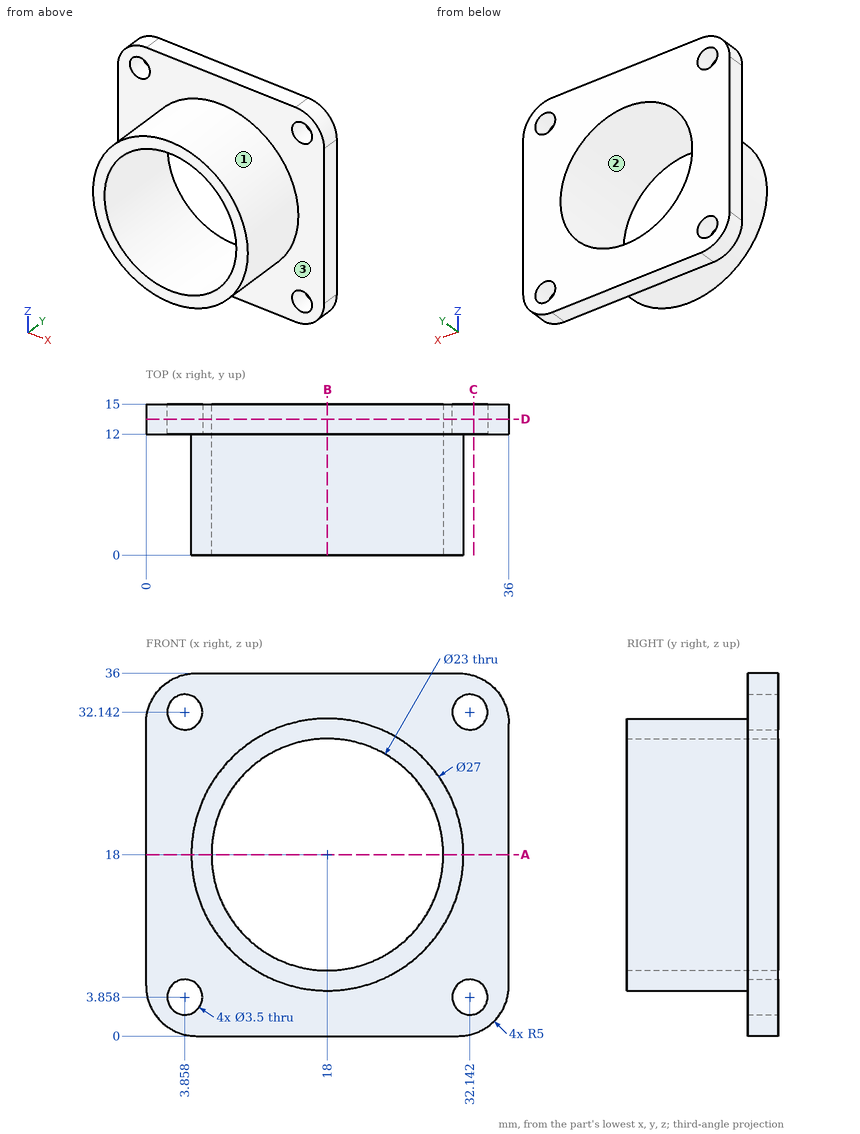
Here's the drawing with two shaded views (mm, measured from the low corner). I have some questions. Round coordinates to 2 decimals unless told otherwise and drop trailing zeros. Order: outer loops, then holes, each group sorted by start corner. A loop starts at its lowest first (then second) coordinate and runs counter-clockwise, first axis right, second up. Notation, with made-up numbers: M 39,9.5 L 72,9.5 A30 ccw 72,37.5 Z; hole C 69,6 d7. An arc over 180 degrees is marked long. Use CSV: the item, a comma, the result in double quotes.
1) I'm going to push flat-ended pins straight in: P1, Ø3, axis at x = 17, y = 8.5, coming from the -Z side; P2, Ø20.5, axis at x = 18, z = 18, coming from the -Y side; P3, Ø6, axis at x = 30, y = 2, coming from the +Z side. Where does each tip first touch, or does it pass through?
Taken from the geometry:
P1,"z = 4.5"
P2,"through"
P3,"z = 28.06"
2) I want a section at B-B (x = 18). List the corners of the cut face in (y, z) for me, then the cut area to 3 significant figures.
Taken from the geometry:
outline,"M 0,4.5 L 12,4.5 L 12,0 L 15,0 L 15,6.5 L 0,6.5 Z; M 0,29.5 L 15,29.5 L 15,36 L 12,36 L 12,31.5 L 0,31.5 Z"
area,"87.0 mm^2"
3) I need wall thicknesses on line 1 along Y through (x, z) = (3.5, 7); line 2 along Z through (x, y) = (3, 13); line 3 along X through (y, z) = (13.25, 10). Which ranges of each line are inside material? Lowest first, please. Write a range as [from, to].
Taken from the geometry:
line 1,"[12, 15]"
line 2,"[0.42, 2.33], [5.38, 30.62], [33.67, 35.58]"
line 3,"[0, 9.74], [26.26, 36]"
4) If we mould it in two halves opening along X, with no side actions, what happens to the marked faces 1, 2 and 3? For each: pulls with the +X half, pulls with the -X half, needs draft (parallel to the pull), parting line crosses it, or undercut.
Taken from the geometry:
face 1,"parting line crosses it"
face 2,"undercut"
face 3,"needs draft"
5) I want a section at A-A (z = 18). List the corners of the cut face in (x, y) for me, then the cut area to 3 significant figures.
Taken from the geometry:
outline,"M 0,12 L 4.5,12 L 4.5,0 L 6.5,0 L 6.5,15 L 0,15 Z; M 29.5,0 L 31.5,0 L 31.5,12 L 36,12 L 36,15 L 29.5,15 Z"
area,"87.0 mm^2"
6) I want a section at C-C (x = 32.5). List the corners of the cut face in (y, z) for me (1 decimal).
Taken from the geometry:
outline,"M 12,0.2 L 15,0.2 L 15,2.1 L 12,2.1 Z; M 12,5.6 L 15,5.6 L 15,30.4 L 12,30.4 Z; M 12,33.9 L 15,33.9 L 15,35.8 L 12,35.8 Z"
7) I want a section at D-D (y = 13.5). List the corners of the cut face in (x, z) for me, then the cut area to 3 significant figures.
Taken from the geometry:
outline,"M 0,5 A5 ccw 5,0 L 31,0 A5 ccw 36,5 L 36,31 A5 ccw 31,36 L 5,36 A5 ccw 0,31 Z; hole C 3.86,3.86 d3.5; hole C 3.86,32.14 d3.5; hole C 18,18 d23; hole C 32.14,3.86 d3.5; hole C 32.14,32.14 d3.5"
area,"821 mm^2"
